The listing builds one solid part. Answer for the finished solid, in the listing's coordinates (mm). A direction names the side the tool comes from. Coordinates: 2 decimals unless noted, no trailing zeros. Write each loop counter-clockwise with the first axis right and the second up, starting at its lowest first coordinate (ties: lowest second). Pieces come first, ordered by that corner, then holes. Notation, with made-up numbers: M -10.5,14 L 26.5,14 A8 ccw 26.5,28 Z; hole C 70,24 d2. An arc over 180 degrees is marked long. Answer as CSV lines item,"result".
```python
from build123d import *

# Parameters (mm, degrees)
F0_W          = 5
F0_H          = 10.2
F0_W_2        = 6.7
F1_DEPTH      = 5
F2_DEPTH      = 1
F4_DEPTH      = 2.5
F4_DEPTH_BACK = 0.8


with BuildPart() as f1:
    # F0 (on Top) → F1 (new body)
    with BuildSketch(Plane.XY):
        with Locations((9.2, -0.2)):
            Rectangle(F0_W, F0_H)
        with Locations((3.35, -0.2)):
            Rectangle(F0_W_2, F0_H)
    extrude(amount=F1_DEPTH)

    # F0 (on Top) → F2 (join)
    with BuildSketch(Plane.XY):
        with Locations((9.2, -0.2)):
            Rectangle(F0_W, F0_H)
    extrude(amount=-F2_DEPTH)

    # F3 (on face) → F4 (join, two sides)
    with BuildSketch(Plane(origin=(0, 0, 0), x_dir=(0, -1, 0), z_dir=(-1, 0, 0))) as f4_sk:
        with BuildLine():
            ThreePointArc((2.0396078054, 0), (2.7494384351, 0.9997549034), (3, 2.2))
            ThreePointArc((3, 2.2), (2.4729636961, 3.8983670268), (1.0770329614, 5))
            Line((1.0770329614, 5), (-1.0770329614, 5))
            ThreePointArc((-1.0770329614, 5), (-2.9459060435, 2.7671310101), (-2.0396078054, 0))
            Line((-2.0396078054, 0), (2.0396078054, 0))
        make_face()
        with BuildLine():
            Line((-1.0770329614, 5), (1.0770329614, 5))
            ThreePointArc((1.0770329614, 5), (0, 5.2), (-1.0770329614, 5))
        make_face()
        with BuildLine():
            ThreePointArc((-2.0396078054, 0), (0, -0.8), (2.0396078054, 0))
            Line((2.0396078054, 0), (-2.0396078054, 0))
        make_face()
    extrude(amount=F4_DEPTH)
    extrude(f4_sk.sketch, amount=-F4_DEPTH_BACK)


solid = f1.part
```
Q1. Straight lines are drawn through the part: line 1 (Z direction, x = 1.25, y = 0.5); line 2 (X direction, y = -2.25, z = 4.75); line 3 (Z direction, x = 11, y = 2.5). For each, find the intervals that lie inside material, in ascending order.
Output:
line 1,"0 to 5"
line 2,"0 to 11.7"
line 3,"-1 to 5"
Q2. Find section A-A (z = 4). Give the vertices of the cut face in (x, y).
Output:
outline,"M -2.5,-2.4 L 0,-2.4 L 0,-5.3 L 11.7,-5.3 L 11.7,4.9 L 0,4.9 L 0,2.4 L -2.5,2.4 Z"
Q3. Find section B-B (y = -2.5). Give the vertices of the cut face in (x, z), and give its area (3 significant figures).
Output:
outline,"M -2.5,0.54 L 0,0.54 L 0,0 L 6.7,0 L 6.7,-1 L 11.7,-1 L 11.7,5 L 0,5 L 0,3.86 L -2.5,3.86 Z"
area,"71.8 mm2"
Q4. For faces 4 (the flat face through (6.7, -0.3, -0.5)), 5 (the flat face through (9, 0, -1)), determine the directions among +Z, -Z, +X, -X, +Y, -Y from which every point of the face is accessible in a straight line to the end or side of a thin tool.
Output:
face 4,"-Z, +Y, -Y"
face 5,"-Z, +X, -X, +Y, -Y"
Q5. Flat-ended cylindrical pins translate along their axes: pin 1 Ø1.5 at (x, y) = (-0.5, -3) entering from +Z; pin 2 Ø1.3 at (y, z) = (-4, 2) entering from -X. Find the tip coordinate at first contact, or state that the pin passes through.
Output:
pin 1,"z = 5"
pin 2,"x = 0"
Q6. Find section D-D (z = 1). Give the vertices of the cut face in (x, y), and give its area (3 significant figures).
Output:
outline,"M -2.5,-2.75 L 0,-2.75 L 0,-5.3 L 11.7,-5.3 L 11.7,4.9 L 0,4.9 L 0,2.75 L -2.5,2.75 Z"
area,"133 mm2"
Q7. The mould has two halves that part along X. Classify faces 1 (the flat face through (3, 0, 0)), 2 (the flat face through (6, 0, 5)), 3 (the flat face through (-2.5, 0, 2)): pulls with the +X half, pulls with the -X half, needs draft (parallel to the pull), parting line crosses it, or undercut.
Output:
face 1,"undercut"
face 2,"needs draft"
face 3,"pulls with the -X half"
Q8. Find section C-C (x = 10). Give the vertices of the cut face in (y, z).
Output:
outline,"M -5.3,-1 L 4.9,-1 L 4.9,5 L -5.3,5 Z"
